Could you check a few things on this model? Use its own coordinates, in mm. Face numbers are marked on the shaded views. Round coordinates to 2 decimals unless told otherwise and drop trailing zeros. Order: outer loops, then holes, each group sorted by start corner. A loop starts at its lowest first (then second) coordinate and runs counter-clockwise, first axis right, second up. Notation, with made-up numbers: (78, -5) -> (116, -5) arc R27 ccw to (116, 33) -> close; hole circle Ø5 at (44, -32.5). An arc over 180 degrees is marked (long way). Put each result on its own line as item: value. Start each with the question number.
from build123d import *

# Parameters (mm, degrees)
SKETCH_1_W      = 40
SKETCH_1_H      = 80
SKETCH_1_R      = 5
EXTRUDE_1_DEPTH = 60


with BuildPart() as part:
    # Эскиз1 → Бобышка-Вытянуть1 (new body)
    with BuildSketch(Plane(origin=(0, 0, 0), x_dir=(0, 0, -1), z_dir=(1, 0, 0))):
        with Locations((20, 40)):
            Rectangle(SKETCH_1_W, SKETCH_1_H)
        with Locations((20, 60)):
            Circle(SKETCH_1_R, mode=Mode.SUBTRACT)
        with Locations((20, 20)):
            Circle(SKETCH_1_R, mode=Mode.SUBTRACT)
    extrude(amount=EXTRUDE_1_DEPTH)


solid = part.part
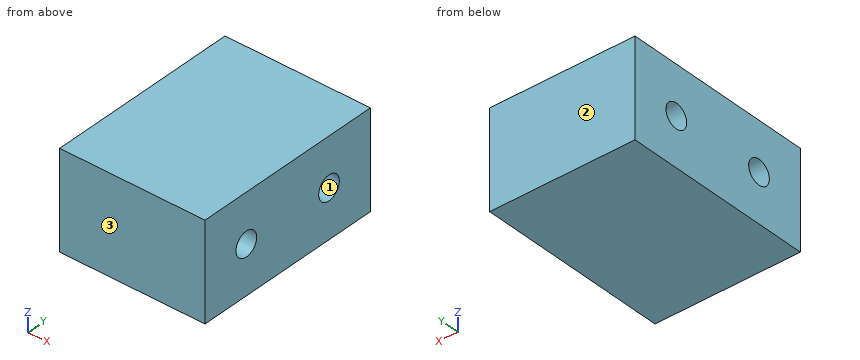
1. If we section it at B-B, the plane y = 60: Please give me the cut outline in (x, z), then the cut area to 3 significant figures.
2. If we section it at C-C, the plane x = 36.5: Please give me the cut outline in (y, z).
3. I need wall thicknesses on L1, parallel to Y at x = 37, z = -20; L2, parallel to Y at x = 56, z = -19; L3, parallel to Z at x = 5.5, y = 61. Which ranges of each line are inside material? Lowest first, please.
4. For pin 1 Ø8 at (y, z) = (20, -20) entering from +X, with a flat end and sliding along its axis, tell me the tip position at first contact or that it passes through.
5. Thinking about a two-plate mould opening in Y: for the marked faces 1, 2 and 3, which applies, +Y half, -Y half, draft (parallel to the pull), parting line (faces both ways), or undercut?
6. If we section it at A-A, the plane z = -20: Please give me the cut outline in (x, y), then the cut area to 3 significant figures.
Results below:
1. outline: (0, -40) -> (60, -40) -> (60, -25) -> (0, -25) -> close; (0, -15) -> (60, -15) -> (60, 0) -> (0, 0) -> close
1. area: 1,800 mm2
2. outline: (0, -40) -> (80, -40) -> (80, 0) -> (0, 0) -> close; hole circle Ø10 at (20, -20); hole circle Ø10 at (60, -20)
3. L1: 0 to 15, 25 to 55, 65 to 80
3. L2: 0 to 15.1, 24.9 to 55.1, 64.9 to 80
3. L3: -40 to -24.9, -15.1 to 0
4. pin 1: through
5. face 1: undercut
5. face 2: +Y half
5. face 3: -Y half
6. outline: (0, 0) -> (60, 0) -> (60, 15) -> (0, 15) -> close; (0, 25) -> (60, 25) -> (60, 55) -> (0, 55) -> close; (0, 65) -> (60, 65) -> (60, 80) -> (0, 80) -> close
6. area: 3,600 mm2
